Could you check a few things on this model? Use its own coordinates, in mm. Face numbers are marked on the shaded views. A direction names the side the tool comes from. Give positions to 0.01 mm unless a question says otherwise; leave off trailing zeros. Order: outer loops, then holes, each group sorted by start corner. A loop starts at its lowest first (then second) coordinate and runs counter-clockwise, first axis right, second up.
(1) Imagine slicing it at B-B, the plane z = 28.25. Write out the boundary of the cut face in (x, y) (3 decimals), then the cut area to 3 significant figures.
(2) Will these pins go through, and if not, where does the flat tip stop? pin 1 (3.5 mm diameter, centred on x = 25.25, z = 13.75, fed in from -Y); pin 2 (8 mm diameter, centred on y = 7, z = 78, fed in from -X); pin 3 (2 mm diameter, centred on x = 5.5, y = 17.5, fed in from +Z); pin 4 (10 mm diameter, centred on y = 9, z = 39, fed in from -X).
(3) Imagine slicing it at C-C, the plane x = 9.75. State how many separate pieces and enclosed holes the cut face has, then the cut area to 3 significant figures.
(4) If I drill on probe 1 along Z at (x, y) = (9.75, 17); probe 2 along Z at (x, y) = (17.5, 14.75); probe 3 along X at (y, z) = (16, 28.25), over which ranges is the centre line in solid material (lowest first)?
(5) Imagine slicing it at A-A, the plane x = 17.5. Write out the boundary of the cut face in (y, z) (3 decimals), then the cut area to 3 significant figures.
(6) On a 3-axis mill with a long thin cutter (end or side, diameter ignored), from which of +Z, -Z, +X, -X, +Y, -Y can I reach the whole of each face in a straight line? I mean the marked faces 1, 2 and 3. Say none if no direction works.
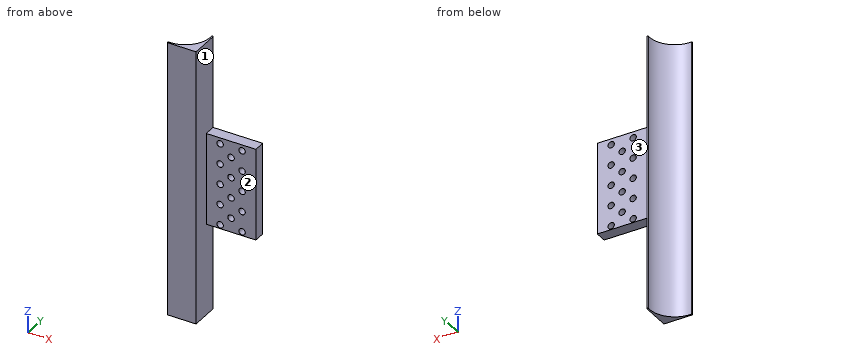
from build123d import *

# Parameters (mm, degrees)
SALIENTE_EXTRUIR1_DEPTH                = 97.5
CROQUIS2_W                             = 65
CROQUIS2_H                             = 8
SALIENTE_EXTRUIR2_DEPTH                = 35
TALADRO_DE_MARGEN_PARA_M41_D           = 4.5
TALADRO_DE_MARGEN_PARA_M41_CSINK_D     = 4.55
TALADRO_DE_MARGEN_PARA_M41_CSINK_ANGLE = 90


with BuildPart() as part:
    # Croquis1 → Saliente-Extruir1 (new, symmetric)
    with BuildSketch(Plane.XY):
        with BuildLine():
            Line((-20, 0), (0, 0))
            Line((0, 0), (0, 20))
            ThreePointArc((0, 20), (-0.513905625, 20.499806596), (-0.999226534, 19.972199507))
            ThreePointArc((-0.999226534, 19.972199507), (-6.24345971, 6.24345971), (-19.972199507, 0.999226534))
            ThreePointArc((-19.972199507, 0.999226534), (-20.499806596, 0.513905625), (-20, 0))
        make_face()
    extrude(amount=SALIENTE_EXTRUIR1_DEPTH, both=True)

    # Croquis2 → Saliente-Extruir2 (add)
    with BuildSketch(Plane(origin=(0, 0, 0), x_dir=(0, 0, -1), z_dir=(1, 0, 0))):
        with Locations((0, 16)):
            Rectangle(CROQUIS2_W, CROQUIS2_H)
    extrude(amount=SALIENTE_EXTRUIR2_DEPTH)

    # Taladro de margen para M41 (through all)
    with Locations(Plane(origin=(0, 12, 0), x_dir=(-1, 0, 0), z_dir=(0, -1, 0))):
        with Locations((-9.75, -28.25), (-25.25, -28.25), (-25.25, -13.75), (-17.5, -21), (-9.75, -13.75), (-9.75, 0.75), (-25.25, 0.75), (-17.5, -6.5), (-17.5, 8), (-9.75, 15.25), (-25.25, 15.25), (-9.75, 29.75), (-17.5, 22.5), (-25.25, 29.75)):
            CounterSinkHole(TALADRO_DE_MARGEN_PARA_M41_D / 2, TALADRO_DE_MARGEN_PARA_M41_CSINK_D / 2, counter_sink_angle=TALADRO_DE_MARGEN_PARA_M41_CSINK_ANGLE)


solid = part.part
Answer block:
1. outline: (-20, 0) - (0, 0) - (0, 12) - (7.475, 12) - (7.5, 12.025) - (7.5, 20) - (0, 20) arc R0.5 ccw (long way) to (-0.999, 19.972) arc R18 cw to (-19.972, 0.999) arc R0.5 ccw (long way) to start; (12, 12.025) - (12.025, 12) - (22.975, 12) - (23, 12.025) - (23, 20) - (12, 20) - close; (27.5, 12.025) - (27.525, 12) - (35, 12) - (35, 20) - (27.5, 20) - close
1. area: 316 mm2
2. pin 1: passes through
2. pin 2: stops at x = -10.67
2. pin 3: stops at z = 32.5
2. pin 4: stops at x = -8.98
3. separate pieces: 6
3. enclosed holes: 0
3. area: 340 mm2
4. probe 1: z = -32.5 to -32, -27.5 to -17.5, -13 to -3, 1.5 to 11.5, 16 to 26, 30.5 to 32.5
4. probe 2: z = -32.5 to -24.75, -20.25 to -10.25, -5.75 to 4.25, 8.75 to 18.75, 23.25 to 32.5
4. probe 3: x = -1.22 to 7.5, 12 to 23, 27.5 to 35
5. outline: (12, -32.5) - (20, -32.5) - (20, -24.75) - (12.025, -24.75) - (12, -24.775) - close; (12, -20.225) - (12.025, -20.25) - (20, -20.25) - (20, -10.25) - (12.025, -10.25) - (12, -10.275) - close; (12, -5.725) - (12.025, -5.75) - (20, -5.75) - (20, 4.25) - (12.025, 4.25) - (12, 4.225) - close; (12, 8.775) - (12.025, 8.75) - (20, 8.75) - (20, 18.75) - (12.025, 18.75) - (12, 18.725) - close; (12, 23.275) - (12.025, 23.25) - (20, 23.25) - (20, 32.5) - (12, 32.5) - close
5. area: 376 mm2
6. face 1: +X, -Y
6. face 2: +Z, -Z, +X, -Y
6. face 3: +Z, -Z, +X, +Y
